Read the model definition and answer for the solid it produces. Units are mm, in the model's axes. Face numbers are marked on the shaded views. A direction names the side the tool comes from. Give positions to 0.01 mm unless a question says otherwise; leave off trailing zeros. Order: outer loops, then holes, each group sorted by start corner. A loop starts at its lowest first (then second) coordinate and runs counter-clockwise, first axis right, second up. Notation, with made-up numbers: (58.5, 68.5) - (100.5, 68.5) arc R20 ccw to (100.5, 101.5) - close; hole circle Ø4 at (-18, 70.5). An arc over 180 degrees is marked (long way). Use a Markdown table: item, result. Add a question column.
1. A cutting plane is placed at C-C on y = -26. Determine the outline of the cut face in (x, z), and give its area (3 significant figures).
2. Consider L1, parallel to Y at x = 4.5, z = 2.5; L2, parallel to Y at x = 21, z = 1; L3, parallel to Z at x = -1, y = -5.5. Determine where each line is inside the solid, lowest interval first.
3. Flat-ended cylindrical pins translate along their axes: P1, Ø1.2, axis at x = 0, z = 3, coming from the -Y side; P2, Ø1.5, axis at y = -12, z = 18, coming from the +X side; P3, Ø2, axis at y = -7.5, z = 4, coming from the +X side. Find the tip coordinate at first contact, or state that the pin passes through.
4. A cutting plane is placed at D-D on z = 3. Determine the outline of the cut face in (x, y).
5. A cutting plane is placed at A-A on x = 0. Determine the outline of the cut face in (y, z), and give its area (3 significant figures).
6. A cutting plane is placed at B-B on z = 10. Determine the outline of the cut face in (x, y), and give its area (3 significant figures).
7. Which of the six approach directions +Z, -Z, +X, -X, +Y, -Y give full straight-line access (tool end or side, diameter ignored) to the marked faces 1 and 2?
```python
from build123d import *

# Parameters (mm, degrees)
BOSS_EXTRU_1_DEPTH      = 4
ENL_V_MAT_EXTRU_1_DEPTH = 50
BOSS_EXTRU_2_DEPTH      = 16
ENL_V_MAT_EXTRU_2_REACH = 64.735
ENL_V_MAT_EXTRU_4_DEPTH = 66.148525236


with BuildPart() as part:
    # Esquisse1 → Boss.-Extru.1 (new body)
    with BuildSketch(Plane.XY):
        with BuildLine():
            Line((-11.273273273, 8.708708709), (34.726726727, 8.708708709))
            ThreePointArc((34.726726727, 8.708708709), (36.140940289, 8.122922271), (36.726726727, 6.708708709))
            Line((36.726726727, 6.708708709), (36.726726727, -9.291291291))
            ThreePointArc((36.726726727, -9.291291291), (36.140940289, -10.705504854), (34.726726727, -11.291291291))
            Line((34.726726727, -11.291291291), (-11.273273273, -11.291291291))
            ThreePointArc((-11.273273273, -11.291291291), (-12.687486836, -10.705504854), (-13.273273273, -9.291291291))
            Line((-13.273273273, -9.291291291), (-13.273273273, 6.708708709))
            ThreePointArc((-13.273273273, 6.708708709), (-12.687486836, 8.122922271), (-11.273273273, 8.708708709))
        make_face()
    extrude(amount=BOSS_EXTRU_1_DEPTH)

    # Esquisse3 → Enlèv. mat.-Extru.1 (cut)
    with BuildSketch(Plane.XY.offset(4)):
        with BuildLine():
            Line((-4.273273273, 1.708708709), (11.726726727, 1.708708709))
            ThreePointArc((11.726726727, 1.708708709), (12.433833508, 1.41581549), (12.726726727, 0.708708709))
            Line((12.726726727, 0.708708709), (12.726726727, -3.291291291))
            ThreePointArc((12.726726727, -3.291291291), (12.433833508, -3.998398072), (11.726726727, -4.291291291))
            Line((11.726726727, -4.291291291), (-4.273273273, -4.291291291))
            ThreePointArc((-4.273273273, -4.291291291), (-4.980380054, -3.998398072), (-5.273273273, -3.291291291))
            Line((-5.273273273, -3.291291291), (-5.273273273, 0.708708709))
            ThreePointArc((-5.273273273, 0.708708709), (-4.980380054, 1.41581549), (-4.273273273, 1.708708709))
        make_face()
    extrude(amount=-ENL_V_MAT_EXTRU_1_DEPTH, mode=Mode.SUBTRACT)

    # Esquisse4 → Boss.-Extru.2 (add)
    with BuildSketch(Plane.XY.offset(4)):
        Polygon((27.400678474, 7.708708709), (51.823328204, -34.592561481), (49.225251993, -36.092561481), (23.359226589, 8.708708709), (25.668627666, 8.708708709), (26.823328204, 8.708708709), align=None)
    extrude(amount=BOSS_EXTRU_2_DEPTH)

    # Esquisse6 → Enlèv. mat.-Extru.2 (cut, up to next)
    with BuildSketch(Plane(origin=(21.29040143, 12.292018997, 0), x_dir=(0, 0, 1), z_dir=(-0.8660254037844363, -0.5000000000000042, 0)), mode=Mode.PRIVATE) as enl_v_mat_extru_2_sk1:
        with BuildLine():
            Line((8, -29.869701126), (12, -29.869701126))
            ThreePointArc((12, -29.869701126), (12.707106781, -30.162594345), (13, -30.869701126))
            Line((13, -30.869701126), (13, -46.869701126))
            ThreePointArc((13, -46.869701126), (12.707106781, -47.576807907), (12, -47.869701126))
            Line((12, -47.869701126), (8, -47.869701126))
            ThreePointArc((8, -47.869701126), (7.292893219, -47.576807907), (7, -46.869701126))
            Line((7, -46.869701126), (7, -30.869701126))
            ThreePointArc((7, -30.869701126), (7.292893219, -30.162594345), (8, -29.869701126))
        make_face()
    enl_v_mat_extru_2_tool1 = extrude(enl_v_mat_extru_2_sk1.sketch, amount=-ENL_V_MAT_EXTRU_2_REACH, mode=Mode.PRIVATE) & part.part
    add(enl_v_mat_extru_2_tool1.solids().sort_by_distance((40.725252, -21.37013, 10))[0], mode=Mode.SUBTRACT)

    # Esquisse11 → Enlèv. mat.-Extru.4 (cut, through all)
    with BuildSketch(Plane.XY.offset(4)):
        with BuildLine():
            Line((36.749431367, 6.794564493), (36.991578009, -8.903216578))
            Line((36.991578009, -8.903216578), (27.400678474, 7.708708709))
            Line((27.400678474, 7.708708709), (26.823328204, 8.708708709))
            Line((26.823328204, 8.708708709), (34.726726727, 8.708708709))
            ThreePointArc((34.726726727, 8.708708709), (36.561329958, 8.621578074), (36.749431367, 6.794564493))
        make_face()
    extrude(amount=-ENL_V_MAT_EXTRU_4_DEPTH, mode=Mode.SUBTRACT)


solid = part.part
```
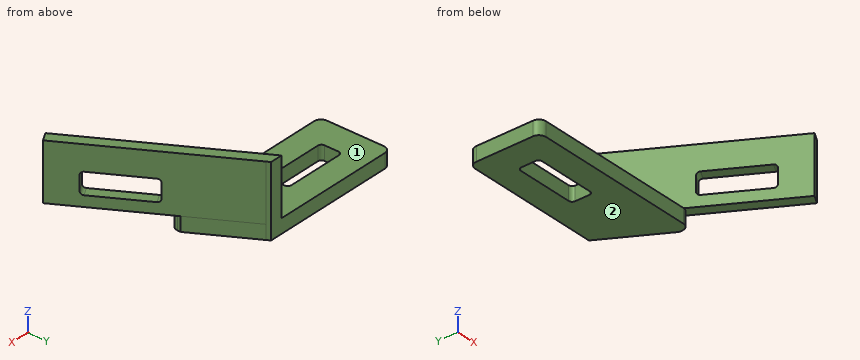
Output values:
| question | item | result |
|---|---|---|
| 1 | outline | (43.4, 4) - (46.86, 4) - (46.86, 7) - (43.4, 7) - close; (43.4, 13) - (46.86, 13) - (46.86, 20) - (43.4, 20) - close |
| 1 | area | 34.6 mm² |
| 2 | L1 | -11.29 to -4.29, 1.71 to 8.71 |
| 2 | L2 | -11.29 to 8.71 |
| 2 | L3 | 0 to 4 |
| 3 | P1 | y = -11.29 |
| 3 | P2 | x = 39.21 |
| 3 | P3 | x = 36.76 |
| 4 | outline | (-13.27, -9.29) arc R2 ccw to (-11.27, -11.29) - (34.73, -11.29) arc R2 ccw to (36.73, -9.29) - (36.73, -8.44) - (26.82, 8.71) - (-11.27, 8.71) arc R2 ccw to (-13.27, 6.71) - close; hole (-5.27, -3.29) arc R1 ccw to (-4.27, -4.29) - (11.73, -4.29) arc R1 ccw to (12.73, -3.29) - (12.73, 0.71) arc R1 ccw to (11.73, 1.71) - (-4.27, 1.71) arc R1 ccw to (-5.27, 0.71) - close |
| 5 | outline | (-11.29, 0) - (-4.29, 0) - (-4.29, 4) - (-11.29, 4) - close; (1.71, 0) - (8.71, 0) - (8.71, 4) - (1.71, 4) - close |
| 5 | area | 56.0 mm² |
| 6 | outline | (23.36, 8.71) - (36.23, -13.58) - (38.82, -12.08) - (26.82, 8.71) - close; (45.23, -29.16) - (49.23, -36.09) - (51.82, -34.59) - (47.82, -27.66) - close |
| 6 | area | 98.6 mm² |
| 7 | face 1 | +Z, -X, -Y |
| 7 | face 2 | -Z, +X, -X, +Y, -Y |
